Could you check a few things on this model? Use its own coordinates, in mm. A direction names the side the tool comes from. Coordinates: 2 decimals unless noted, no trailing zeros. Loops run counter-clockwise (first coordinate to the right, second up) from the corner with the lowest first, then second, coordinate; pieces in that order, holes last.
from build123d import *

# Parameters (mm, degrees)
F0_W     = 44.45
F0_H     = 44.45
F1_DEPTH = 107.95
F3_D     = 12.7


with BuildPart() as f1:
    # F0 (on Top) → F1 (new body)
    with BuildSketch(Plane.XY):
        with BuildLine():
            ThreePointArc((25.4, 22.225), (24.470064, 24.470064), (22.225, 25.4))
            Line((22.225, 25.4), (-22.225, 25.4))
            ThreePointArc((-22.225, 25.4), (-24.470064, 24.470064), (-25.4, 22.225))
            Line((-25.4, 22.225), (-25.4, -22.225))
            ThreePointArc((-25.4, -22.225), (-24.470064, -24.470064), (-22.225, -25.4))
            Line((-22.225, -25.4), (22.225, -25.4))
            ThreePointArc((22.225, -25.4), (24.470064, -24.470064), (25.4, -22.225))
            Line((25.4, -22.225), (25.4, 22.225))
        make_face()
        Rectangle(F0_W, F0_H, mode=Mode.SUBTRACT)
    extrude(amount=F1_DEPTH)

    # F3 (through all)
    with Locations(Plane.YZ.offset(25.4)):
        with Locations((0, 0)):
            Hole(F3_D / 2)


solid = f1.part
(1) I need wall thicknesses on probe 1 along X at (y, z) = (6, 49) (3 decimals); probe 2 along X at (y, z) = (22.5, 79). Which ranges of each line are inside material? Lowest first, please.
Answers:
probe 1: x = -25.4 to -22.225, 22.225 to 25.4
probe 2: x = -25.39 to 25.39
(2) Which directions (+Z, -Z, +X, -X, +Y, -Y) give clear straight access to the entire face, cutting with the end or side of a thin tool? Please do faces 1 (the face through (-25.4, 0, 53)), 2 (the face through (0, -22.225, 53)).
Answers:
face 1: +Z, -Z, -X, +Y, -Y
face 2: +Z, -Z
(3) Imagine slicing it at C-C, the plane z = 51. Write out the boundary of the cut face in (x, y) (3 decimals), and give its area (3 significant figures).
Answers:
outline: (-25.4, -22.225) arc R3.175 ccw to (-22.225, -25.4) - (22.225, -25.4) arc R3.175 ccw to (25.4, -22.225) - (25.4, 22.225) arc R3.175 ccw to (22.225, 25.4) - (-22.225, 25.4) arc R3.175 ccw to (-25.4, 22.225) - close; hole (-22.225, -22.225) - (22.225, -22.225) - (22.225, 22.225) - (-22.225, 22.225) - close
area: 596 mm2
(4) Imagine slicing it at A-A, the plane y = -21. Write out the boundary of the cut face in (x, z) (3 decimals), and give its area (3 significant figures).
Answers:
outline: (-25.4, 0) - (-22.225, 0) - (-22.225, 107.95) - (-25.4, 107.95) - close; (22.225, 0) - (25.4, 0) - (25.4, 107.95) - (22.225, 107.95) - close
area: 685 mm2
(5) We'd pull the mould along X, two halves only. Please class faces 3 (the face through (24.49, 24.45, 53.22)), 4 (the face through (0, 22.225, 53)), 5 (the face through (0, 25.4, 53)): +X half, -X half, draft (parallel to the pull), parting line (faces both ways), or undercut.
Answers:
face 3: +X half
face 4: undercut
face 5: draft
